from build123d import *

# Parameters (mm, degrees)
BOSS_EXTRUDE1_DEPTH   = 6.35
SKETCH3_W             = 12.7
SKETCH3_H             = 6.35
SKETCH3_R             = 1.651
CUT_EXTRUDE2_DEPTH    = 3.175
F_4_40_TAPPED_HOLE1_D = 2.2606
M2_CLEARANCE_HOLE1_D  = 2.6
FILLET1_R             = 3.81


with BuildPart() as part:
    # Sketch1 → Boss-Extrude1 (new body)
    with BuildSketch(Plane(origin=(0, 0, 0), x_dir=(1, 0, 0), z_dir=(0, 1, 0))):
        with BuildLine():
            Line((13.850000078, -23.754236173), (13.850000078, 5.291734921))
            ThreePointArc((13.850000078, 5.291734921), (11.827298987, 12.498502631), (6.35, 17.600268634))
            Line((6.35, 17.600268634), (6.35, 37.56114916))
            ThreePointArc((6.35, 37.56114916), (5.606051224, 39.357200384), (3.81, 40.10114916))
            Line((3.81, 40.10114916), (-3.81, 40.10114916))
            ThreePointArc((-3.81, 40.10114916), (-5.606051224, 39.357200384), (-6.35, 37.56114916))
            Line((-6.35, 37.56114916), (-6.35, 17.600268634))
            ThreePointArc((-6.35, 17.600268634), (-11.827298987, 12.498502631), (-13.850000078, 5.291734921))
            Line((-13.850000078, 5.291734921), (-13.850000078, -23.754236173))
            ThreePointArc((-13.850000078, -23.754236173), (-11.827298987, -30.961003884), (-6.35, -36.062769886))
            Line((-6.35, -36.062769886), (-6.35, -56.023651732))
            ThreePointArc((-6.35, -56.023651732), (-5.606051224, -57.819702956), (-3.81, -58.563651732))
            Line((-3.81, -58.563651732), (3.81, -58.563651732))
            ThreePointArc((3.81, -58.563651732), (5.606051224, -57.819702956), (6.35, -56.023651732))
            Line((6.35, -56.023651732), (6.35, -36.062769886))
            ThreePointArc((6.35, -36.062769886), (11.827298987, -30.961003884), (13.850000078, -23.754236173))
        make_face()
    extrude(amount=BOSS_EXTRUDE1_DEPTH)

    # Sketch3 → Cut-Extrude2 (cut)
    with BuildSketch(Plane.XZ):
        with Locations((0, -23.59114916)):
            Rectangle(SKETCH3_W, SKETCH3_H)
        with Locations((0, -23.59114916)):
            Circle(SKETCH3_R, mode=Mode.SUBTRACT)
        with Locations((0, -23.59114916)):
            Circle(SKETCH3_R)
        with Locations((0, 42.053651732)):
            Rectangle(SKETCH3_W, SKETCH3_H)
        with Locations((0, 42.053651732)):
            Circle(SKETCH3_R, mode=Mode.SUBTRACT)
        with Locations((0, 42.053651732)):
            Circle(SKETCH3_R)
    extrude(amount=-CUT_EXTRUDE2_DEPTH, mode=Mode.SUBTRACT)

    # #4-40 Tapped Hole1 (through all)
    with Locations(Plane(origin=(0, 0, 0), x_dir=(-1, 0, 0), z_dir=(0, -1, 0))):
        with Locations((0, -52.213651732), (0, 33.75114916)):
            Hole(F_4_40_TAPPED_HOLE1_D / 2)

    # M2 Clearance Hole1 (through all)
    with Locations(Plane(origin=(0, 0, 0), x_dir=(-1, 0, 0), z_dir=(0, -1, 0))):
        with Locations((9.50000005, 5.291734921), (0, 14.791734971), (-9.50000005, 5.291734921), (0, -4.208265129)):
            Hole(M2_CLEARANCE_HOLE1_D / 2)

    # Fillet1
    fillet1_edges = [part.edges().sort_by_distance(p)[0] for p in [
        (-6.35, 3.175, 36.062769886),
        (-6.35, 3.175, -17.600268634),
        (6.35, 3.175, -17.600268634),
        (6.35, 3.175, 36.062769886),
    ]]
    fillet(fillet1_edges, radius=FILLET1_R)


solid = part.part
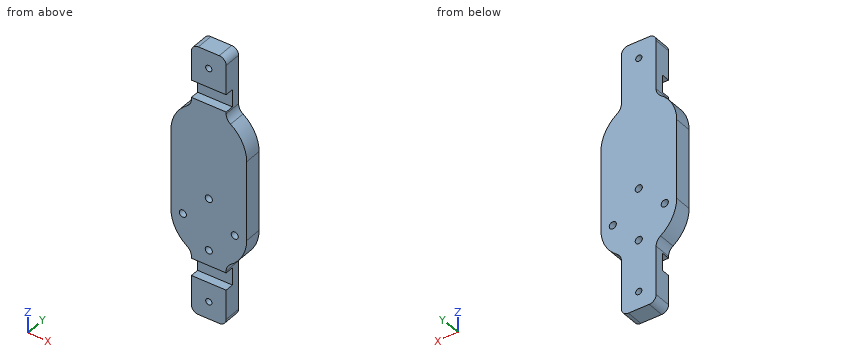
The listing builds one solid part. Answer for the finished solid, in the listing's coordinates (mm). Give positions to 0.01 mm unless a question says otherwise; leave off trailing zeros. Write each loop counter-clockwise with the first axis right and the second up, starting at its lowest first coordinate (ties: lowest second). Pieces come first, ordered by that corner, then holes.
Item 1: Section B-B, the plane y = 2 is taken. Count the separate pieces of the cut face and the enclosed holes in it, plus the area to 3 significant figures.
Item 2: Section D-D, the plane z = 41 is taken. Write down the section's boundary in (x, y) (3 decimals), plus the area to 3 significant figures.
Item 3: Find the intervals of material crossed by line 1 along Z through (x, y) = (-1.5, 2.75); line 2 along Z through (x, y) = (0, 3.5); line 3 along X through (y, z) = (4.75, -5.5), in increasing order.
Item 4: Flat-ended cylindrical pins translate along their axes: P1, Ø6, axis at x = -10.5, z = -12, coming from the -Y side; P2, Ø2, axis at x = 0, z = -14.79, coming from the +Y side; P3, Ø2, axis at x = 5, y = 4, coming from the -Z side; P4, Ø1.9, axis at y = 4, z = -29.5, coming from the +X side. Find the tip coordinate at first contact, or state that the pin passes through.
Item 5: Section A-A, the plane x = 0 is taken. Write down the section's boundary in (y, z) (3 decimals), plus the area to 3 significant figures.
Item 6: Section C-C, the plane x = -9.5 is taken. Write down the section's boundary in (y, z).
Completed:
1. separate pieces: 3
1. enclosed holes: 6
1. area: 1,760 mm2
2. outline: (-6.35, 3.175) - (6.35, 3.175) - (6.35, 6.35) - (-6.35, 6.35) - close
2. area: 40.3 mm2
3. line 1: z = -40.1 to -26.77, -20.42 to 38.88, 45.23 to 58.56
3. line 2: z = -40.1 to -34.88, -32.62 to -16.09, -13.49 to 2.91, 5.51 to 51.08, 53.34 to 58.56
3. line 3: x = -13.85 to -10.78, -8.22 to 8.22, 10.78 to 13.85
4. P1: stops at y = 0
4. P2: passes through
4. P3: stops at z = -40.09
4. P4: stops at x = 6.35
5. outline: (0, -40.101) - (6.35, -40.101) - (6.35, -34.881) - (0, -34.881) - close; (0, -32.621) - (6.35, -32.621) - (6.35, -16.092) - (0, -16.092) - (0, -20.416) - (3.175, -20.416) - (3.175, -26.766) - (0, -26.766) - close; (0, -13.492) - (6.35, -13.492) - (6.35, 2.908) - (0, 2.908) - close; (0, 5.508) - (6.35, 5.508) - (6.35, 51.083) - (0, 51.083) - (0, 45.229) - (3.175, 45.229) - (3.175, 38.879) - (0, 38.879) - close; (0, 53.344) - (6.35, 53.344) - (6.35, 58.564) - (0, 58.564) - close
5. area: 524 mm2
6. outline: (0, -15.37) - (6.35, -15.37) - (6.35, -6.59) - (0, -6.59) - close; (0, -3.99) - (6.35, -3.99) - (6.35, 33.83) - (0, 33.83) - close
